from build123d import *


with BuildPart() as part:
    # Sketch1 → Revolve1 (revolve)
    with BuildSketch(Plane.XY):
        with BuildLine():
            Line((26.680645161, 2), (26.680645161, 0))
            Line((26.680645161, 0), (21.680645161, 0))
            Line((21.680645161, 0), (21.680645161, 2.5))
            Line((21.680645161, 2.5), (-13.319354839, 2.5))
            Line((-13.319354839, 2.5), (-13.294296878, 8.9999517))
            ThreePointArc((-13.294296878, 8.9999517), (-10.365170466, 13.062306261), (-5.383476734, 12.547297834))
            ThreePointArc((-5.383476734, 12.547297834), (-3.084370729, 11.035442519), (-0.656411636, 9.740602932))
            Line((-0.656411636, 9.740602932), (21.680645161, 9.740602932))
            ThreePointArc((21.680645161, 9.740602932), (25.216179067, 8.276136838), (26.680645161, 4.740602932))
            Line((26.680645161, 4.740602932), (26.680645161, 2))
        make_face()
    revolve(axis=Axis((-16.009165471, 0, 0), (1, 0, 0)))


solid = part.part
Verification items for the finished model (mm, model axes). Coordinates: 2 decimals unless noted, no trailing zeros. Order: outer loops, then holes, each group sorted by start corner. A loop starts at its lowest first (then second) coordinate and runs counter-clockwise, first axis right, second up. Notation, with made-up numbers: M 40,44.5 L 98,44.5 A24 ccw 98,76.5 Z; hole C 36.25,29.5 d11. An arc over 180 degrees is marked long. Write each question's results on one line, items separated by ' | '.
1) Section check A-A on x = -9. Record the cut outline in (y, z), plus the area to 3 significant figures.
Solved:
outline: C 0,0 d26.91; hole C 0,0 d5 | area: 549 mm²
2) Gauge pin test, flat ends, axial feed: pin 1 Ø2 at (x, y) = (-4.5, -4.5) entering from +Z; pin 2 Ø1.5 at (x, y) = (-4, 8) entering from +Z; pin 3 Ø1 at (x, y) = (2, -4) entering from -Z. Record the tip position at first contact, or that the pin passes through.
Solved:
pin 1: stops at z = 11.88 | pin 2: stops at z = 9.33 | pin 3: stops at z = -9.09
3) Section check B-B on x = -4.5. Record the cut outline in (y, z).
Solved:
outline: C 0,0 d23.86; hole C 0,0 d5
4) Release check for a two-part mould opening along Y. For faces 1 (the face through (10.67, -2.11, -9.51)), 2 (the face through (3.94, -0.54, -2.44)), 3 (the face through (21.681, 0, 0)), 4 (the face through (26.681, 0, 0)) record: pulls with the +Y half, pulls with the -Y half, needs draft (parallel to the pull), parting line crosses it, or undercut.
Solved:
face 1: parting line crosses it | face 2: undercut | face 3: undercut | face 4: needs draft
5) Scan lines: line 1 along Z through (x, y) = (6, 0); line 2 along Y through (x, z) = (16, -1.25); line 3 along X through (y, z) = (0.75, 2). Record each from-to range of solid material in increasing order. Write a range as [from, to].
Solved:
line 1: z = [-9.74, -2.5], [2.5, 9.74] | line 2: y = [-9.66, -2.17], [2.17, 9.66] | line 3: x = [21.68, 26.68]
